For this review, use the dimensioned drawing (mm, ordinates from the lowest corner) and the shaded views. A direction names the side the tool comes from. Coordinates: 2 decimals unless noted, no trailing zeros. Order: outer loops, then holes, each group sorted by start corner. A loop starts at its lowest first (then second) coordinate and runs counter-clockwise, first axis right, second up. Notation, with made-up numbers: M 12,49.5 L 32,49.5 A27 cw 32,68.5 Z; hole C 57,-7.75 d5. An arc over 180 degrees is marked long. Write each question's results on one line, items separated by ' | '.
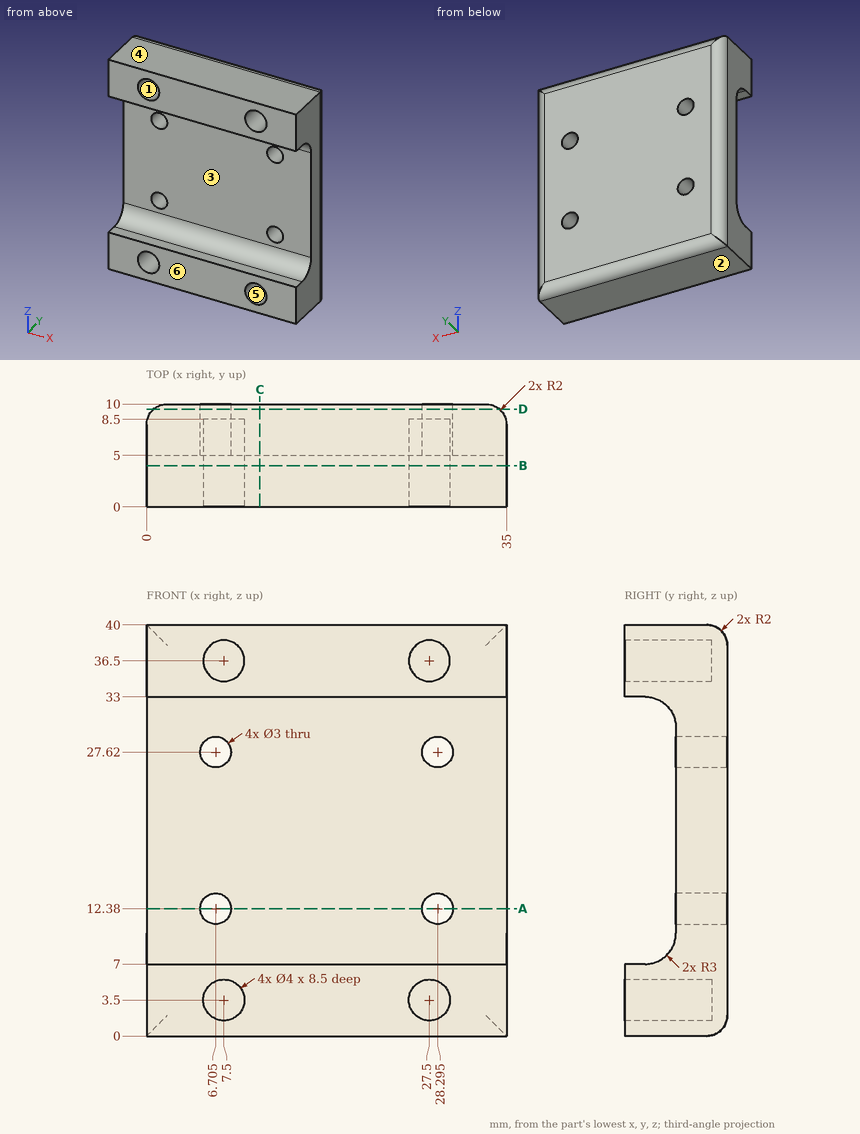
1) Take a section at B-B on y = 4. State the section outline as (x, z) points.
Solutions:
outline: M 0,0 L 35,0 L 35,7.76 L 0,7.76 Z; M 0,32.24 L 35,32.24 L 35,40 L 0,40 Z; hole C 7.5,3.5 d4; hole C 7.5,36.5 d4; hole C 27.5,3.5 d4; hole C 27.5,36.5 d4
2) Take a section at C-C on x = 11. State the section outline as (y, z) points, plus the area to 3 significant figures.
Solutions:
outline: M 0,0 L 8,0 A2 ccw 10,2 L 10,38 A2 ccw 8,40 L 0,40 L 0,33 L 2,33 A3 cw 5,30 L 5,10 A3 cw 2,7 L 0,7 Z | area: 272 mm2
3) For pin 1 (3 mm diameter, centred on x = 7.5, z = 3.5, fed in from -Y); pin 2 (4.5 mm diameter, centred on x = 7.5, z = 4, fed in from -Y); pin 3 (5 mm diameter, centred on x = 6.705, z = 27.62, fed in from -Y), all flat-tipped, find the tip position at first contact; note any pin that passes through.
Solutions:
pin 1: y = 8.5 | pin 2: y = 0 | pin 3: y = 5
4) The part is to be moulded in two halves that separate along Z. For the marked faces 4, 5 and 6, say which applies: pulls with the +Z half, pulls with the -Z half, needs draft (parallel to the pull), parting line crosses it, or undercut.
Solutions:
face 4: pulls with the +Z half | face 5: undercut | face 6: needs draft
5) For the marked faces 1, 2 and 3, list the 3-axis set-ups (+Z, -Z, +X, -X, +Y, -Y) from which the entire face can be reached by the end or side of a thin tool; tool diameter is ignored.
Solutions:
face 1: -Y | face 2: -Z, +X, -X, +Y, -Y | face 3: +X, -X, -Y
6) To check wall thickness, follow line 1 along X through (y, z) = (7.45, 12.38) (3 decimals); line 2 along X through (y, z) = (4, 36.5); line 3 along Z through (x, y) = (26, 6.75). State the ranges of each line that lie inside material, in increasing order.
Solutions:
line 1: 0 to 5.205, 8.205 to 26.795, 29.795 to 35 | line 2: 0 to 5.5, 9.5 to 25.5, 29.5 to 35 | line 3: 0 to 2.18, 4.82 to 35.18, 37.82 to 40
7) Take a section at A-A on z = 12.38. State the section outline as (x, y) points (3 decimals), plus the area to 3 significant figures.
Solutions:
outline: M 0,5 L 5.205,5 L 5.205,10 L 2,10 A2 ccw 0,8 Z; M 8.205,5 L 26.795,5 L 26.795,10 L 8.205,10 Z; M 29.795,5 L 35,5 L 35,8 A2 ccw 33,10 L 29.795,10 Z | area: 143 mm2
8) Take a section at D-D on y = 9.5. State the section outline as (x, z) points (3 decimals).
Solutions:
outline: M 0.677,0.677 L 34.323,0.677 L 34.323,39.323 L 0.677,39.323 Z; hole C 6.705,12.38 d3; hole C 6.705,27.62 d3; hole C 28.295,12.38 d3; hole C 28.295,27.62 d3
